Source: CAD feature listing. Evaluate the final solid. Frame: model axes, mm. A direction names the side the tool comes from. Round coordinates to 2 decimals unless told otherwise and drop trailing zeros. Loops run counter-clockwise (first coordinate to the right, second up) from the corner with the lowest first, then second, coordinate; pieces in that order, holes last.
Item 1: Section query C-C on z = -4.75. Return loops of the section in (x, y).
Item 2: Ray query, L1, parallel to Y at x = 33.5, z = 3; L2, parallel to Z at x = -28.5, y = 71; L3, parallel to Y at x = -18.5, z = -16.5. Return the intervals inside material, ascending.
Item 3: Pull-direction query (Y, two-part tool) for faces 1 (the flat face through (3, 77.495, 2)), 2 (the flat face through (37, 38.433, 2)), 3 (the flat face through (39, -47.505, 2)); classes: released by +Y, released by -Y, zero draft, split by the parting line, or undercut.
Item 4: Access query for faces 4 (the flat face through (26, -20, -20)), 5 (the cylindrical face through (-16.15, -16.38, -9.86)), 6 (the flat face through (-33, -38.927, 2)). Directions: +Z, -Z, +X, -X, +Y, -Y. A direction counts if a zero-diameter tool reaches every point of the face in a straight line with its end or side. Return the directions, or none.
Item 5: Section query B-B on x = -24. Return loops of the section in (y, z), then the cut area to 3 significant figures.
Item 6: Section query A-A on y = 47. Return loops of the section in (x, z), then the cut area to 3 significant figures.
Item 7: Section query D-D on y = -6.5. Return loops of the section in (x, z), then the cut area to 3 significant figures.
Item 8: First-contact query: P1, Ø1.7, axis at x = -18.93, y = 73.5, coming from the -Z side; P2, Ø6, axis at x = 7.5, y = -43, coming from the -Z side; P3, Ø10, axis at x = 30.5, z = -8.5, coming from the +Y side; P4, Ø12, axis at y = -32, z = -2, coming from the -X side. Flat tips, straight axial feed; report the tip coordinate or a pass-through.
```python
from build123d import *

# Parameters (mm, degrees)
F4_R            = 3.5
F5_DEPTH        = 4
F6_D            = 2.5
F6_CBORE_D      = 4.5
F6_CBORE_DEPTH  = 2
F7_DEPTH        = 20
F9_D            = 2.9
F9_DEPTH        = 18
F9_CSINK_D      = 4
F9_CSINK_ANGLE  = 90
F9_TIP          = 0.8712478976
F11_D           = 2.9
F11_DEPTH       = 18
F11_CSINK_D     = 4
F11_CSINK_ANGLE = 90
F11_TIP         = 0.8712478976
F13_D           = 2.9
F13_DEPTH       = 18
F13_CSINK_D     = 4
F13_CSINK_ANGLE = 90
F13_TIP         = 0.8712478976
F15_D           = 2.9
F15_DEPTH       = 18
F15_CSINK_D     = 4
F15_CSINK_ANGLE = 90
F15_TIP         = 0.8712478976
F16_DEPTH       = 25
F18_DEPTH       = 25
F19_DEPTH       = 25
F20_W           = 20
F20_H           = 30.4843550548
F20_H_2         = 31.25
F20_H_3         = 30.620081059
F21_DEPTH       = 4
F17_R           = 7.5
F22_DEPTH       = 4
F23_W           = 43
F23_H           = 4
F24_DEPTH       = 10
F26_D           = 2.5
F26_DEPTH       = 15
F26_CSINK_D     = 4
F26_CSINK_ANGLE = 90
F26_TIP         = 0.7510757738
F27_D           = 2.5
F27_DEPTH       = 15
F27_CSINK_D     = 4
F27_CSINK_ANGLE = 90
F27_TIP         = 0.7510757738


with BuildPart() as f5:
    # F4 (on Top) → F5 (new body)
    with BuildSketch(Plane.XY):
        Polygon((27.5709562153, 77.495081059), (-22.4290437847, 77.495081059), (-22.4290437847, 73.495081059), (-22.4290437847, -18.5049188996), (-22.4290437847, -22.504918941), (27.5709562153, -22.504918941), (27.5709562153, -18.504918941), (27.5709562153, 73.495081059), align=None)
        with BuildLine():
            ThreePointArc((-15.4290437847, -18.504918941), (-18.9290438054, -22.004918941), (-22.4290437847, -18.5049188996))
            ThreePointArc((-22.4290437847, -18.5049188996), (-18.9290437641, -15.004918941), (-15.4290437847, -18.504918941))
        make_face(mode=Mode.SUBTRACT)
        with Locations((24.0709562153, -18.504918941)):
            Circle(F4_R, mode=Mode.SUBTRACT)
        with BuildLine():
            ThreePointArc((-15.4290437847, 73.495081059), (-18.9290437847, 69.995081059), (-22.4290437847, 73.495081059))
            ThreePointArc((-22.4290437847, 73.495081059), (-18.9290437847, 76.995081059), (-15.4290437847, 73.495081059))
        make_face(mode=Mode.SUBTRACT)
        with Locations((24.0709562153, 73.495081059)):
            Circle(F4_R, mode=Mode.SUBTRACT)
        with BuildLine():
            ThreePointArc((-15.4290437847, -18.504918941), (-18.9290437641, -15.004918941), (-22.4290437847, -18.5049188996))
            ThreePointArc((-22.4290437847, -18.5049188996), (-18.9290438054, -22.004918941), (-15.4290437847, -18.504918941))
        make_face()
        with Locations((24.0709562153, -18.504918941)):
            Circle(F4_R)
        with BuildLine():
            ThreePointArc((-15.4290437847, 73.495081059), (-18.9290437847, 76.995081059), (-22.4290437847, 73.495081059))
            ThreePointArc((-22.4290437847, 73.495081059), (-18.9290437847, 69.995081059), (-15.4290437847, 73.495081059))
        make_face()
        with Locations((24.0709562153, 73.495081059)):
            Circle(F4_R)
    extrude(amount=F5_DEPTH)

    # F6 (through all)
    with Locations(Plane(origin=(0, 0, 0), x_dir=(1, 0, 0), z_dir=(0, 0, -1))):
        with Locations((19.7709562153, -69.995081059), (19.7709562153, 15.004918941), (-14.6290437847, 15.004918941), (-14.6290437847, -69.995081059)):
            CounterBoreHole(F6_D / 2, F6_CBORE_D / 2, F6_CBORE_DEPTH)

    # F4 (on Top) → F7 (join)
    with BuildSketch(Plane.XY):
        with BuildLine():
            ThreePointArc((-15.4290437847, -18.504918941), (-18.9290437641, -15.004918941), (-22.4290437847, -18.5049188996))
            ThreePointArc((-22.4290437847, -18.5049188996), (-18.9290438054, -22.004918941), (-15.4290437847, -18.504918941))
        make_face()
        with Locations((24.0709562153, -18.504918941)):
            Circle(F4_R)
        with BuildLine():
            ThreePointArc((-15.4290437847, 73.495081059), (-18.9290437847, 76.995081059), (-22.4290437847, 73.495081059))
            ThreePointArc((-22.4290437847, 73.495081059), (-18.9290437847, 69.995081059), (-15.4290437847, 73.495081059))
        make_face()
        with Locations((24.0709562153, 73.495081059)):
            Circle(F4_R)
    extrude(amount=-F7_DEPTH)

    # F9
    with Locations(Plane(origin=(0, 0, -20), x_dir=(1, 0, 0), z_dir=(0, 0, -1))):
        with Locations((-18.9290437847, -73.495081059)):
            CounterSinkHole(F9_D / 2, F9_CSINK_D / 2, depth=F9_DEPTH, counter_sink_angle=F9_CSINK_ANGLE)
            with Locations((0, 0, -(F9_DEPTH + F9_TIP / 2))):  # 118° drill point
                Cone(0, F9_D / 2, F9_TIP, mode=Mode.SUBTRACT)

    # F11
    with Locations(Plane(origin=(0, 0, -20), x_dir=(1, 0, 0), z_dir=(0, 0, -1))):
        with Locations((-18.9290437847, 18.504918941)):
            CounterSinkHole(F11_D / 2, F11_CSINK_D / 2, depth=F11_DEPTH, counter_sink_angle=F11_CSINK_ANGLE)
            with Locations((0, 0, -(F11_DEPTH + F11_TIP / 2))):  # 118° drill point
                Cone(0, F11_D / 2, F11_TIP, mode=Mode.SUBTRACT)

    # F13
    with Locations(Plane(origin=(0, 0, -20), x_dir=(1, 0, 0), z_dir=(0, 0, -1))):
        with Locations((24.0709562153, -73.495081059)):
            CounterSinkHole(F13_D / 2, F13_CSINK_D / 2, depth=F13_DEPTH, counter_sink_angle=F13_CSINK_ANGLE)
            with Locations((0, 0, -(F13_DEPTH + F13_TIP / 2))):  # 118° drill point
                Cone(0, F13_D / 2, F13_TIP, mode=Mode.SUBTRACT)

    # F15
    with Locations(Plane(origin=(0, 0, -20), x_dir=(1, 0, 0), z_dir=(0, 0, -1))):
        with Locations((24.0709562153, 18.504918941)):
            CounterSinkHole(F15_D / 2, F15_CSINK_D / 2, depth=F15_DEPTH, counter_sink_angle=F15_CSINK_ANGLE)
            with Locations((0, 0, -(F15_DEPTH + F15_TIP / 2))):  # 118° drill point
                Cone(0, F15_D / 2, F15_TIP, mode=Mode.SUBTRACT)

    # F16 (add): a face of the model
    f16_faces = [f5.faces().sort_by_distance(p)[0] for p in [
        (2.5709562153, -22.504918941, 2),
    ]]
    extrude(f16_faces, amount=F16_DEPTH)

    # F18 (add): a face of the model
    f18_faces = [f5.faces().sort_by_distance(p)[0] for p in [
        (27.5709562153, 14.995081059, 2),
    ]]
    extrude(f18_faces, amount=F18_DEPTH)

    # F19 (add): a face of the model
    f19_faces = [f5.faces().sort_by_distance(p)[0] for p in [
        (-22.4290437847, 14.995081059, 2),
    ]]
    extrude(f19_faces, amount=F19_DEPTH)

    # F20 (on face) → F21 (cut)
    with BuildSketch(Plane.XY.offset(4)):
        with Locations((-32.4290437847, -23.6845964684)):
            Rectangle(F20_W, F20_H)
        with Locations((-32.4290437847, 14.995081059)):
            Rectangle(F20_W, F20_H_2)
        with Locations((-32.4290437847, 54.057581059)):
            Rectangle(F20_W, F20_H_2)
        with Locations((37.5709562153, 54.057581059)):
            Rectangle(F20_W, F20_H_2)
        with Locations((37.5709562153, 15.3100405295)):
            Rectangle(F20_W, F20_H_3)
        with Locations((37.5709562153, -24.067418941)):
            Rectangle(F20_W, F20_H_2)
    extrude(amount=-F21_DEPTH, mode=Mode.SUBTRACT)

    # F17 (on face) → F22 (cut)
    with BuildSketch(Plane.XY.offset(4)):
        with Locations((-7.4290437847, -32.2756583249)):
            Circle(F17_R)
        with Locations((12.5709562153, -32.2756583249)):
            Circle(F17_R)
    extrude(amount=-F22_DEPTH, mode=Mode.SUBTRACT)

    # F23 (on face) → F24 (join)
    with BuildSketch(Plane.XZ.offset(47.504918941)):
        with Locations((2.5709562153, 2)):
            Rectangle(F23_W, F23_H)
    extrude(amount=F24_DEPTH)

    # F26
    with Locations(Plane(origin=(0, 0, 0), x_dir=(1, 0, 0), z_dir=(0, 0, -1))):
        with Locations((2.5709562153, 52.504918941), (2.5709562153, 42.504918941)):
            CounterSinkHole(F26_D / 2, F26_CSINK_D / 2, depth=F26_DEPTH, counter_sink_angle=F26_CSINK_ANGLE)
            with Locations((0, 0, -(F26_DEPTH + F26_TIP / 2))):  # 118° drill point
                Cone(0, F26_D / 2, F26_TIP, mode=Mode.SUBTRACT)

    # F27
    with Locations(Plane(origin=(0, 0, 0), x_dir=(1, 0, 0), z_dir=(0, 0, -1))):
        with Locations((-18.9290437847, 42.504918941), (-18.9290437847, 32.504918941), (24.0709562153, 32.504918941), (24.0709562153, 42.504918941)):
            CounterSinkHole(F27_D / 2, F27_CSINK_D / 2, depth=F27_DEPTH, counter_sink_angle=F27_CSINK_ANGLE)
            with Locations((0, 0, -(F27_DEPTH + F27_TIP / 2))):  # 118° drill point
                Cone(0, F27_D / 2, F27_TIP, mode=Mode.SUBTRACT)


solid = f5.part
```
Data:
1. outline: circle Ø7 at (-18.93, -18.5); circle Ø7 at (-18.93, 73.5); circle Ø7 at (24.07, -18.5); circle Ø7 at (24.07, 73.5); hole circle Ø2.9 at (-18.93, -18.5); hole circle Ø2.9 at (-18.93, 73.5); hole circle Ø2.9 at (24.07, -18.5); hole circle Ø2.9 at (24.07, 73.5)
2. L1: y = -47.5 to -39.69, -8.44 to 0, 30.62 to 38.43, 69.68 to 77.5
2. L2: z = 0 to 4
2. L3: y = -21.98 to -19.89, -17.12 to -15.03, 70.02 to 72.11, 74.88 to 76.97
3. face 1: released by +Y
3. face 2: undercut
3. face 3: released by -Y
4. face 4: -Z, +X, -X, +Y, -Y
4. face 5: -Z
4. face 6: +Z, -Z
5. outline: (-47.5, 0) - (-38.93, 0) - (-38.93, 4) - (-47.5, 4) - close; (-8.44, 0) - (-0.63, 0) - (-0.63, 4) - (-8.44, 4) - close; (30.62, 0) - (38.43, 0) - (38.43, 4) - (30.62, 4) - close; (69.68, 0) - (77.5, 0) - (77.5, 4) - (69.68, 4) - close
5. area: 128 mm2
6. outline: (-47.43, 0) - (-42.43, 0) - (-42.43, 4) - (-47.43, 4) - close; (-22.43, 0) - (27.57, 0) - (27.57, 4) - (-22.43, 4) - close; (47.57, 0) - (52.57, 0) - (52.57, 4) - (47.57, 4) - close
6. area: 240 mm2
7. outline: (-47.43, 0) - (52.57, 0) - (52.57, 4) - (-47.43, 4) - close
7. area: 400 mm2
8. P1: stops at z = -1.64
8. P2: stops at z = 0
8. P3: stops at y = 76.69
8. P4: stops at x = -47.43
